```python
from build123d import *

# Parameters (mm, degrees)
F0_W     = 8.128
F0_H     = 8.128
F1_DEPTH = 17.78
F2_W     = 4.445
F2_H     = 2.54
F3_DEPTH = 25.4
F4_R     = 3.302
F5_DEPTH = 25.4


with BuildPart() as f1:
    # F0 (on Top) → F1 (new body)
    with BuildSketch(Plane.XY):
        with Locations((4.064, 4.064)):
            Rectangle(F0_W, F0_H)
    extrude(amount=F1_DEPTH)

    # F2 (on face) → F3 (cut)
    with BuildSketch(Plane.YZ.offset(8.128)):
        with Locations((5.9055, 15.24)):
            Rectangle(F2_W, F2_H)
    extrude(amount=-F3_DEPTH, mode=Mode.SUBTRACT)

    # F4 (on face) → F5 (cut)
    with BuildSketch(Plane.XZ):
        with Locations((4.064, 10.16)):
            Circle(F4_R)
    extrude(amount=-F5_DEPTH, mode=Mode.SUBTRACT)


solid = f1.part
```
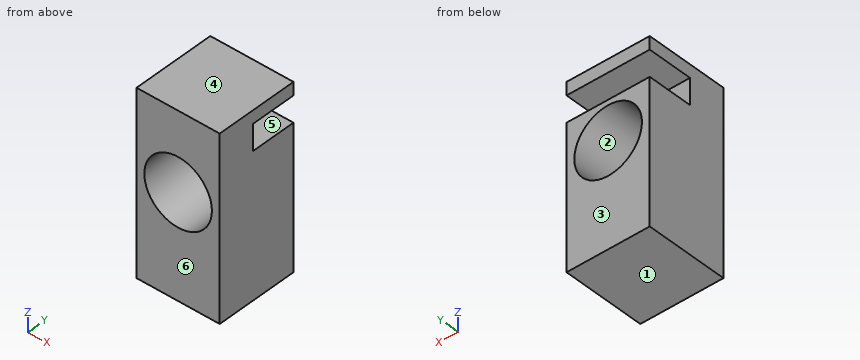
CAD build for the part. Positions are in the model's coordinates, mm. Face numbers are marked on the shaded views. A direction names the side the tool comes from. Coordinates: 2 decimals unless noted, no trailing zeros. Write each loop counter-clockwise with the first axis right and the second up, starting at its lowest first coordinate (ties: lowest second). Pieces come first, ordered by that corner, then holes. Notation, with made-up numbers: (-0.75, -7.75) -> (37.25, -7.75) arc R20 ccw to (37.25, 3.25) -> close; hole circle Ø7 at (80, 8.5). An arc over 180 degrees is marked (long way). Use CSV: the item, a comma, the result in double quotes. Start each with the question number.
Item 1: Tool access for the marked faces 5 and 6: list every direction of +Z, -Z, +X, -X, +Y, -Y with a clear straight run to the whole face (end or side of a thin tool).
Item 2: Band-saw the part on B-B, the plane y = 1. Write the cut outline in (x, z), plus the area to 3 significant figures.
Item 3: Band-saw the part on A-A, the plane z = 10.16. Write the cut outline in (x, y).
Item 4: Wall check: probe 1 along Z at (x, y) = (7.5, 7); probe 2 along Z at (x, y) = (4.75, 7.75); probe 3 along Z at (x, y) = (7, 4.5). Give the ranges that are in metal, low to high.
Item 5: Drop flat-ended pins along their axis: P1, Ø4, axis at x = 1.5, z = 15, coming from the +Y side; P2, Ø2, axis at x = 5, z = 10.5, coming from the -Y side. Give the stop position or say it passes through.
Item 6: Two-plate mould, pull along Z, no slides. Class the marked faces 1, 2, 3 and 4: +Z half, -Z half, draft (parallel to the pull), parting line (faces both ways), or undercut.
Item 7: Band-saw the part on C-C, the plane x = 7. Write the cut outline in (y, z).
Item 8: Band-saw the part on D-D, the plane x = 1.75. Write the cut outline in (y, z).
Response values:
1,face 5,"+X, -X, +Y"
1,face 6,"+Z, -Z, +X, -X, -Y"
2,outline,"(0, 0) -> (8.13, 0) -> (8.13, 17.78) -> (0, 17.78) -> close; hole circle Ø6.6 at (4.06, 10.16)"
2,area,"110 mm2"
3,outline,"(0, 0) -> (0.76, 0) -> (0.76, 8.13) -> (0, 8.13) -> close; (7.37, 0) -> (8.13, 0) -> (8.13, 8.13) -> (7.37, 8.13) -> close"
4,probe 1,"z = 0 to 13.97, 16.51 to 17.78"
4,probe 2,"z = 0 to 6.93, 13.39 to 13.97, 16.51 to 17.78"
4,probe 3,"z = 0 to 8.65, 11.67 to 13.97, 16.51 to 17.78"
5,P1,"stops at y = 8.13"
5,P2,"passes through"
6,face 1,"-Z half"
6,face 2,"undercut"
6,face 3,"draft"
6,face 4,"+Z half"
7,outline,"(0, 0) -> (8.13, 0) -> (8.13, 8.65) -> (0, 8.65) -> close; (0, 11.67) -> (8.13, 11.67) -> (8.13, 13.97) -> (3.68, 13.97) -> (3.68, 16.51) -> (8.13, 16.51) -> (8.13, 17.78) -> (0, 17.78) -> close"
8,outline,"(0, 0) -> (8.13, 0) -> (8.13, 7.8) -> (0, 7.8) -> close; (0, 12.52) -> (8.13, 12.52) -> (8.13, 13.97) -> (3.68, 13.97) -> (3.68, 16.51) -> (8.13, 16.51) -> (8.13, 17.78) -> (0, 17.78) -> close"
